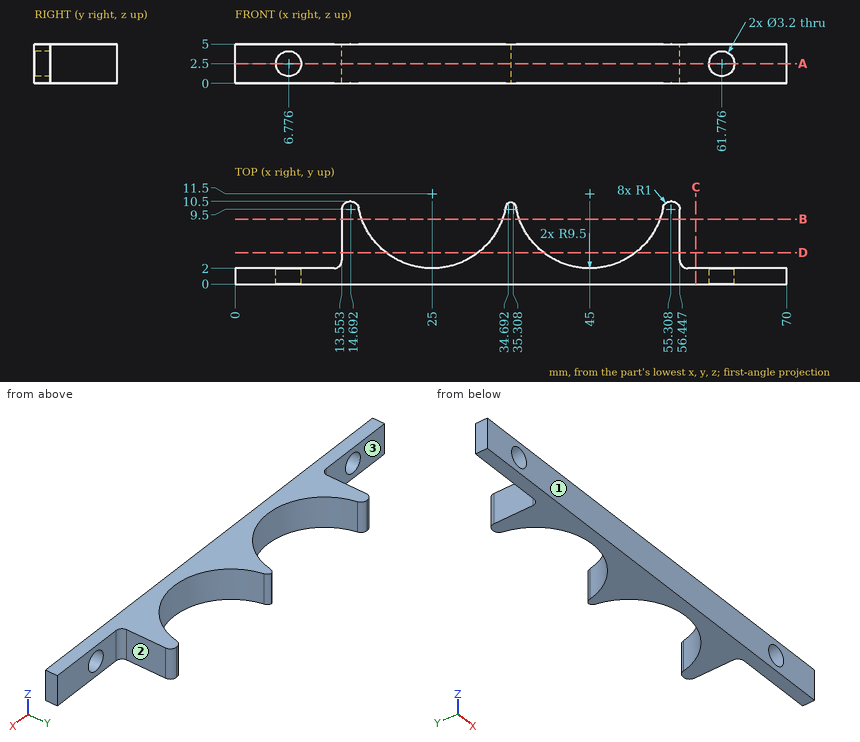
Design review of the part shown in the three views and the two pictorial views. Dimensions are in mm from the part's minimum x, y and z. A direction names the side the tool comes from. Coordinates: 2 decimals unless noted, no trailing zeros. Write each loop counter-clockwise with the first axis right and the second up, starting at its lowest first coordinate (ties: lowest second). Pieces come first, ordered by that corner, then holes.
(1) For pin 1 Ø1.5 at (y, z) = (5, 1.5) entering from -X; pin 2 Ø2.5 at (y, z) = (7.5, 2) entering from +X, all flat-tipped, find the tip position at first contact; note any pin that passes through.
(2) Add section B-B on y = 8.25. Give the boundary of the cut face in (x, z).
(3) Add section D-D on y = 4. Give the boundary of the cut face in (x, z).
(4) Add section C-C on x = 58.5. Give the boundary of the cut face in (y, z), then the cut area to 3 significant figures.
(5) Wall thickness on probe 1 along X at (y, z) = (6, 2.9) (1 decimal); probe 2 along X at (y, z) = (7.5, 1.15); probe 3 along Y at (x, z) = (45.5, 1.65): over which ranges is each line inside the solid? List them lowest first.
(6) Add section A-A on z = 2.5. Give the boundary of the cut face in (x, y).
(7) Tool access review of the marked faces 1, 2 and 3: name each direction out of +Z, -Z, +X, -X, +Y, -Y from which nothing blocks a thin tool from reaching the whole face with its end or side.
Answer sheet:
1. pin 1: stops at x = 13.55
1. pin 2: stops at x = 56.45
2. outline: (13.55, 0) - (16.07, 0) - (16.07, 5) - (13.55, 5) - close; (33.93, 0) - (36.07, 0) - (36.07, 5) - (33.93, 5) - close; (53.93, 0) - (56.45, 0) - (56.45, 5) - (53.93, 5) - close
3. outline: (13.55, 0) - (19.17, 0) - (19.17, 5) - (13.55, 5) - close; (30.83, 0) - (39.17, 0) - (39.17, 5) - (30.83, 5) - close; (50.83, 0) - (56.45, 0) - (56.45, 5) - (50.83, 5) - close
4. outline: (0, 0) - (2, 0) - (2, 5) - (0, 5) - close
4. area: 10.0 mm2
5. probe 1: x = 13.6 to 17.3, 32.7 to 37.3, 52.7 to 56.4
5. probe 2: x = 13.55 to 16.38, 33.62 to 36.38, 53.62 to 56.45
5. probe 3: y = 0 to 2.01
6. outline: (0, 0) - (5.18, 0) - (5.18, 2) - (0, 2) - close; (8.38, 0) - (60.18, 0) - (60.18, 2) - (57.45, 2) arc R1 cw to (56.45, 3) - (56.45, 9.5) arc R1 ccw to (55.45, 10.5) - (55.31, 10.5) arc R1 ccw to (54.33, 9.69) arc R9.5 cw to (35.67, 9.69) arc R1 ccw to (35, 10.45) arc R1 ccw to (34.33, 9.69) arc R9.5 cw to (15.67, 9.69) arc R1 ccw to (14.69, 10.5) - (14.55, 10.5) arc R1 ccw to (13.55, 9.5) - (13.55, 3) arc R1 cw to (12.55, 2) - (8.38, 2) - close; (63.38, 0) - (70, 0) - (70, 2) - (63.38, 2) - close
7. face 1: +Z, -Z, +X, -X, -Y
7. face 2: +Z, -Z, +X, +Y
7. face 3: +Z, -Z, -X, +Y
